from build123d import *

# Parameters (mm, degrees)
F0_R          = 3.5
F1_DEPTH      = 3
F0_W          = 6
F0_H          = 150
F2_DEPTH      = 103
F2_DEPTH_BACK = 3
F4_DEPTH      = 25
F5_R          = 3
F6_DEPTH      = 25


with BuildPart() as f1:
    # F0 (on Top) → F1 (new body, symmetric)
    with BuildSketch(Plane.XY):
        with BuildLine():
            Line((-8.5, 17.5), (-8.5, 0))
            Line((-8.5, 0), (-8.5, -17.5))
            ThreePointArc((-8.5, -17.5), (-2.642136, -31.642136), (11.5, -37.5))
            Line((11.5, -37.5), (41.5, -37.5))
            Line((41.5, -37.5), (73.142136, -69.142136))
            ThreePointArc((73.142136, -69.142136), (79.630603, -73.477591), (87.284271, -75))
            Line((87.284271, -75), (381.5, -75))
            Line((381.5, -75), (381.5, 75))
            Line((381.5, 75), (87.284271, 75))
            ThreePointArc((87.284271, 75), (79.630603, 73.477591), (73.142136, 69.142136))
            Line((73.142136, 69.142136), (41.5, 37.5))
            Line((41.5, 37.5), (11.5, 37.5))
            ThreePointArc((11.5, 37.5), (-2.642136, 31.642136), (-8.5, 17.5))
        make_face()
        Circle(F0_R, mode=Mode.SUBTRACT)
    extrude(amount=F1_DEPTH, both=True)

    # F0 (on Top) → F2 (join, two sides)
    with BuildSketch(Plane.XY) as f2_sk:
        with Locations((384.5, 0)):
            Rectangle(F0_W, F0_H)
    extrude(amount=F2_DEPTH)
    extrude(f2_sk.sketch, amount=-F2_DEPTH_BACK)

    # F3 (on face) → F4 (cut)
    with BuildSketch(Plane(origin=(381.5, 0, 0), x_dir=(0, -1, 0), z_dir=(-1, 0, 0))):
        with BuildLine():
            ThreePointArc((27.5, 53), (0, 80.5), (-27.5, 53))
            ThreePointArc((-27.5, 53), (0, 25.5), (27.5, 53))
        make_face()
        with BuildLine():
            ThreePointArc((55, 103), (69.142136, 97.142136), (75, 83))
            Line((75, 83), (75, 103))
            Line((75, 103), (55, 103))
        make_face()
        with BuildLine():
            Line((-75, 103), (-75, 83))
            ThreePointArc((-75, 83), (-69.142136, 97.142136), (-55, 103))
            Line((-55, 103), (-75, 103))
        make_face()
        with BuildLine():
            Line((-27.5, 103), (-47.5, 103))
            ThreePointArc((-47.5, 103), (-33.357864, 97.142136), (-27.5, 83))
            Line((-27.5, 83), (-27.5, 53))
            ThreePointArc((-27.5, 53), (0, 80.5), (27.5, 53))
            Line((27.5, 53), (27.5, 83))
            ThreePointArc((27.5, 83), (33.357864, 97.142136), (47.5, 103))
            Line((47.5, 103), (32.5, 103))
            Line((32.5, 103), (-27.5, 103))
        make_face()
    extrude(amount=-F4_DEPTH, mode=Mode.SUBTRACT)

    # F5 (on face) → F6 (cut)
    with BuildSketch(Plane.XY.offset(3)):
        with Locations((159.392136, 70)):
            Circle(F5_R)
        with Locations((309.392136, 70)):
            Circle(F5_R)
        with Locations((309.392136, -70)):
            Circle(F5_R)
        with Locations((159.392136, -70)):
            Circle(F5_R)
    extrude(amount=-F6_DEPTH, mode=Mode.SUBTRACT)


solid = f1.part
Verification items for the finished model (mm, model axes). A direction names the side the tool comes from. Round coordinates to 2 decimals unless told otherwise and drop trailing zeros. Loops run counter-clockwise (first coordinate to the right, second up) from the corner with the lowest first, then second, coordinate; pieces in that order, holes last. Notation, with made-up numbers: (-21, -19) - (0, -19) arc R9 cw to (0, -3) - close; hole circle Ø7 at (-15.5, 6). An arc over 180 degrees is marked (long way). Use one line per item in the form item = value.
1. Section check A-A on y = 0. Record the cut outline in (x, z).
A:
outline = (-8.5, -3) - (-3.5, -3) - (-3.5, 3) - (-8.5, 3) - close; (3.5, -3) - (387.5, -3) - (387.5, 25.5) - (381.5, 25.5) - (381.5, 3) - (3.5, 3) - close
2. Access from +Z, -Z, +X, -X, +Y, -Y to the whole of each face (thin tool, end or side, straight path). Record for faces 4 (the flat face through (184, 1, 3)), 5 (the cylindrical face through (384.458, -68.986, 97.297)), 6 (the cylindrical face through (384.458, -33.203, 96.986)).
A:
face_4 = +Z, -X, +Y, -Y
face_5 = +Z, +X, -X, -Y
face_6 = +Z, +X, -X
3. Section check C-C on y = 42. Record the cut outline in (x, z).
A:
outline = (46, -3) - (387.5, -3) - (387.5, 102.23) - (381.5, 102.23) - (381.5, 3) - (46, 3) - close
4. Draft check along Y on faces 1 (the cylindrical face through (-2.797, -31.486, 0.042)), 2 (the cylindrical face through (384.458, 33.514, 97.297)), 3 (the flat face through (387.5, -18, 27)). Enter one of: pulls with the +Y half, pulls with the -Y half, needs draft (parallel to the pull), parting line crosses it, or undercut.
A:
face_1 = pulls with the -Y half
face_2 = undercut
face_3 = needs draft
5. Section check D-D on x = 111. Record the cut outline in (y, z).
A:
outline = (-75, -3) - (75, -3) - (75, 3) - (-75, 3) - close
6. Scan lines: probe 1 along X at (y, z) = (64, 35); probe 2 along Z at (x, y) = (272.5, -20); probe 3 along Y at (x, z) = (0, 0). Record each from-to range of solid material in increasing order.
A:
probe_1 = 381.5 to 387.5
probe_2 = -3 to 3
probe_3 = -33.86 to -3.5, 3.5 to 33.86
7. Section check B-B on z = 72. Record the cut outline in (x, y), and give its area (3 significant figures).
A:
outline = (381.5, -75) - (387.5, -75) - (387.5, -27.5) - (381.5, -27.5) - close; (381.5, 27.5) - (387.5, 27.5) - (387.5, 75) - (381.5, 75) - close
area = 570 mm²
8. Gauge pin test, flat ends, axial feed: pin 1 Ø1.8 at (x, z) = (30, -1.5) entering from +Y; pin 2 Ø5 at (x, z) = (19.5, 1) entering from -Y; pin 3 Ø1.5 at (x, y) = (171.5, -14.5) entering from +Z. Record the tip position at first contact, or that the pin passes through.
A:
pin_1 = 37.5
pin_2 = -37.5
pin_3 = 3
